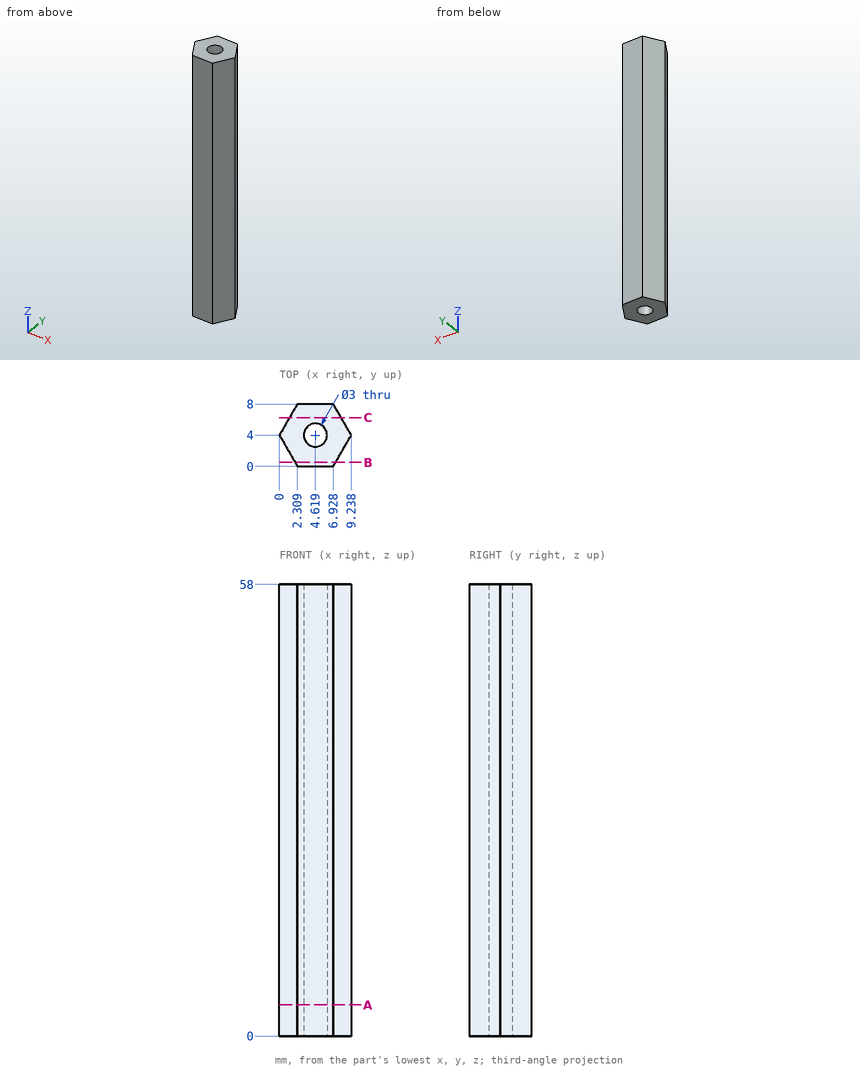
Could you check a few things on this drawing? It's one solid part, dimensions in mm from its lowest x, y, z. Round coordinates to 2 decimals unless told otherwise and drop trailing zeros. Order: outer loops, then holes, each group sorted by start corner. A loop starts at its lowest first (then second) coordinate and runs counter-clockwise, first axis right, second up.
Q1. Imagine slicing it at C-C, the plane y = 6.25. List the corners of the cut face in (x, z) for me.
Geometry says:
outline: (1.3, 0) - (7.94, 0) - (7.94, 58) - (1.3, 58) - close
Q2. Please list where these lines run through material, in increasing order: probe 1 along X at (y, z) = (4, 24); probe 2 along Y at (x, z) = (4.75, 14) (1 decimal); probe 3 along Y at (x, z) = (3.75, 38).
Geometry says:
probe 1: x = 0 to 3.12, 6.12 to 9.24
probe 2: y = 0 to 2.5, 5.5 to 8
probe 3: y = 0 to 2.78, 5.22 to 8
Q3. I'm going to push flat-ended pins straight in: P1, Ø2.5, axis at x = 4.62, y = 4, coming from the +Z side; P2, Ø1, axis at x = 8, z = 8, coming from the -Y side. Where does each tip first touch, or does it pass through?
Geometry says:
P1: passes through
P2: stops at y = 0.99
Q4. Imagine slicing it at A-A, the plane z = 4. List the corners of the cut face in (x, y) for me.
Geometry says:
outline: (0, 4) - (2.31, 0) - (6.93, 0) - (9.24, 4) - (6.93, 8) - (2.31, 8) - close; hole circle Ø3 at (4.62, 4)
Q5. Imagine slicing it at B-B, the plane y = 0.5. List the corners of the cut face in (x, z) for me.
Geometry says:
outline: (2.02, 0) - (7.22, 0) - (7.22, 58) - (2.02, 58) - close
